```python
from build123d import *

# Parameters (mm, degrees)
BOSS_EXTRUDE1_DEPTH = 4
SKETCH2_R           = 1.5
CUT_EXTRUDE1_DEPTH  = 19.874586088
BOSS_EXTRUDE2_DEPTH = 5
SKETCH4_W           = 6
SKETCH4_H           = 6
CUT_EXTRUDE2_DEPTH  = 14
SKETCH6_R           = 1.5
CUT_EXTRUDE3_DEPTH  = 20.111514854
FILLET1_R           = 10
FILLET2_R           = 2
FILLET3_R           = 2


with BuildPart() as part:
    # Sketch1 → Boss-Extrude1 (new, symmetric)
    with BuildSketch(Plane.XY):
        Polygon((2.5, 15.5), (5, 15.5), (5, -15.5), (-5, -15.5), (-5, 15.5), (-2.5, 15.5), (-2.5, 6.5), (2.5, 6.5), align=None)
    extrude(amount=BOSS_EXTRUDE1_DEPTH, both=True)

    # Sketch2 → Cut-Extrude1 (cut, through all)
    with BuildSketch(Plane(origin=(5, 0, 0), x_dir=(0, 0, -1), z_dir=(1, 0, 0))):
        with Locations((0, 12.5)):
            Circle(SKETCH2_R)
    extrude(amount=-CUT_EXTRUDE1_DEPTH, mode=Mode.SUBTRACT)

    # Sketch3 → Boss-Extrude2 (add, symmetric)
    with BuildSketch(Plane(origin=(0, 0, 0), x_dir=(0, 0, -1), z_dir=(1, 0, 0))):
        Polygon((-4, -15.5), (-10, -15.5), (-10, -13.5), (-4, -7.5), align=None)
        Polygon((4, -7.5), (4, -15.5), (10, -15.5), (10, -13.5), align=None)
    extrude(amount=BOSS_EXTRUDE2_DEPTH, both=True)

    # Sketch4 → Cut-Extrude2 (cut)
    with BuildSketch(Plane(origin=(0, 0, 0), x_dir=(1, 0, 0), z_dir=(0, 1, 0))):
        with Locations((0, 7)):
            Rectangle(SKETCH4_W, SKETCH4_H)
        with Locations((0, -7)):
            Rectangle(SKETCH4_W, SKETCH4_H)
    extrude(amount=-CUT_EXTRUDE2_DEPTH, mode=Mode.SUBTRACT)

    # Sketch6 → Cut-Extrude3 (cut, through all)
    with BuildSketch(Plane(origin=(0, 0, 0), x_dir=(1, 0, 0), z_dir=(0, 1, 0))):
        with Locations(Location((0, 7, 0), (0, 0, 270))):
            Circle(SKETCH6_R)
        with Locations(Location((0, -7, 0), (0, 0, 270))):
            Circle(SKETCH6_R)
    extrude(amount=-CUT_EXTRUDE3_DEPTH, mode=Mode.SUBTRACT)

    # Fillet1
    fillet1_edges = [part.edges().sort_by_distance(p)[0] for p in [
        (4, -7.5, 4),
        (4, -7.5, -4),
        (-4, -7.5, -4),
        (-4, -7.5, 4),
    ]]
    fillet(fillet1_edges, radius=FILLET1_R)

    # Fillet2
    fillet2_edges = [part.edges().sort_by_distance(p)[0] for p in [
        (-2.5, 6.5, 0),
        (2.5, 6.5, 0),
    ]]
    fillet(fillet2_edges, radius=FILLET2_R)

    # Fillet3
    fillet3_edges = [part.edges().sort_by_distance(p)[0] for p in [
        (3.75, 15.5, -4),
        (-3.75, 15.5, 4),
        (3.75, 15.5, 4),
        (-3.75, 15.5, -4),
    ]]
    fillet(fillet3_edges, radius=FILLET3_R)


solid = part.part
```
Design review of the part built by this model. Coordinates are the model's own, in mm. A direction names the side the tool comes from. Coordinates: 2 decimals unless noted, no trailing zeros. Order: outer loops, then holes, each group sorted by start corner. A loop starts at its lowest first (then second) coordinate and runs counter-clockwise, first axis right, second up. Notation, with made-up numbers: (-23, 27) - (3, 27) arc R15 cw to (3, 43) - close; hole circle Ø9 at (69, -26). An arc over 180 degrees is marked (long way). Answer in a Markdown table with one row per item.
(1) Consider section A-A on z = 0. State the section outline as (x, y) points.
Checked values:
| item | result |
|---|---|
| outline | (-5, -15.5) - (5, -15.5) - (5, 11) - (2.5, 11) - (2.5, 8.5) arc R2 cw to (0.5, 6.5) - (-0.5, 6.5) arc R2 cw to (-2.5, 8.5) - (-2.5, 11) - (-5, 11) - close; (-5, 14) - (-2.5, 14) - (-2.5, 15.5) - (-5, 15.5) - close; (2.5, 14) - (5, 14) - (5, 15.5) - (2.5, 15.5) - close |
(2) The part is to be moulded in two halves that separate along X. For faces 4 (the flat face through (-3, -11, -6)), 5 (the cylindrical face through (-1.93, 7.1, 0.06)), 6 (the flat face through (-5, -3, 0)), 7 (the cylindrical face through (-4.014, -7.235, -4.782)), say which applies: released by +X, released by -X, zero draft, split by the parting line, or undercut.
Checked values:
| item | result |
|---|---|
| face 4 | undercut |
| face 5 | undercut |
| face 6 | released by -X |
| face 7 | zero draft |
(3) Consider section D-D on z = 6. State the section outline as (x, y) points, plus the area to 3 significant figures.
Checked values:
| item | result |
|---|---|
| outline | (-5, -15.5) - (-1.12, -15.5) - (-1.12, -14) - (-3, -14) - (-3, -9.36) - (-5, -9.36) - close; (1.12, -15.5) - (5, -15.5) - (5, -9.36) - (3, -9.36) - (3, -14) - (1.12, -14) - close |
| area | 30.2 mm^2 |
(4) For faces 1 (the cylindrical face through (1.9, 7.07, 0.06)), 2 (the flat face through (0, 0, -4)), 3 (the flat face through (-3, -11, 6)), list the 3-axis set-ups (+Z, -Z, +X, -X, +Y, -Y) from which the entire face can be reached by the end or side of a thin tool; tool diameter is ignored.
Checked values:
| item | result |
|---|---|
| face 1 | +Z, -Z, +Y |
| face 2 | -Z, +Y |
| face 3 | +Z, +Y |
(5) Consider section C-C on x = 0. State the section outline as (y, z) points, plus the area to 3 significant figures.
Checked values:
| item | result |
|---|---|
| outline | (-15.5, -10) - (-14, -10) - (-14, -8.5) - (-15.5, -8.5) - close; (-15.5, -5.5) - (-14, -5.5) - (-14, -4) - (6.5, -4) - (6.5, 4) - (-14, 4) - (-14, 5.5) - (-15.5, 5.5) - close; (-15.5, 8.5) - (-14, 8.5) - (-14, 10) - (-15.5, 10) - close |
| area | 185 mm^2 |
(6) Consider section B-B on y = 12.5. State the section outline as (x, z) points.
Checked values:
| item | result |
|---|---|
| outline | (-5, -4) - (-2.5, -4) - (-2.5, -1.5) - (-5, -1.5) - close; (-5, 1.5) - (-2.5, 1.5) - (-2.5, 4) - (-5, 4) - close; (2.5, -4) - (5, -4) - (5, -1.5) - (2.5, -1.5) - close; (2.5, 1.5) - (5, 1.5) - (5, 4) - (2.5, 4) - close |
(7) Wall thickness on line 1 along X through (y, z) = (-14.45, 7); line 2 along X through (y, z) = (14.5, 1.5); line 3 along Y through (x, z) = (3.8, 0): over which ranges is each line inside the solid? List them lowest first. Write a range as from..to.
Checked values:
| item | result |
|---|---|
| line 1 | -5..-1.5, 1.5..5 |
| line 2 | -5..-2.5, 2.5..5 |
| line 3 | -15.5..11, 14..15.5 |
(8) Clearance check with flat-ended pins moving along their axes: pin 1 (1.8 mm diameter, centred on y = -6.5, z = -7.5, fed in from +X); pin 2 (0.8 mm diameter, centred on x = 0, z = -1.5, fed in from +Y); pin 3 (1.5 mm diameter, centred on x = 1.5, y = 4, fed in from -Z); pin 4 (1.5 mm diameter, centred on x = -2, y = -4.5, fed in from +Z). State where each tip first meets the part, or that it passes through.
Checked values:
| item | result |
|---|---|
| pin 1 | through |
| pin 2 | y = 6.5 |
| pin 3 | z = -4 |
| pin 4 | z = 4 |
